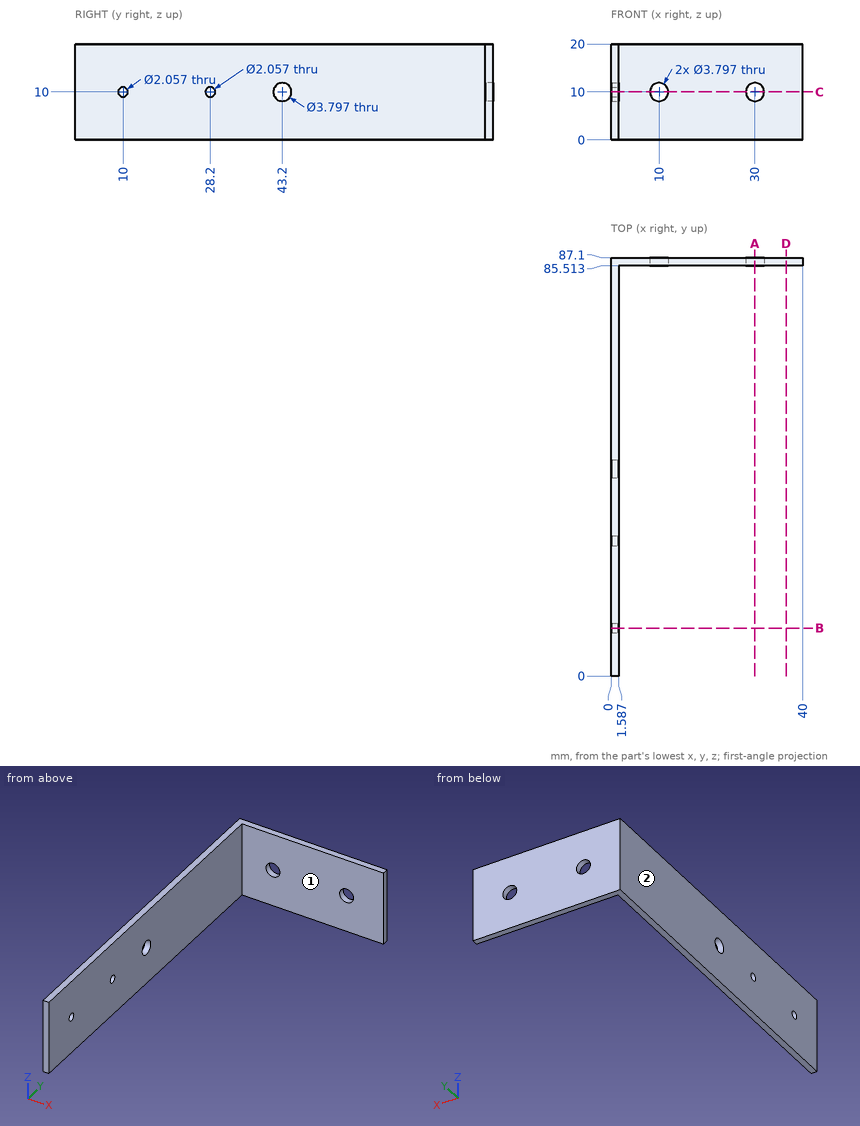
Check sheet for the drawn part. Datum: minimum x, y, z corner. Units: mm. A direction names the side the tool comes from. Coordinates: 2 decimals unless noted, no trailing zeros. Order: outer loops, then holes, each group sorted by start corner. A loop starts at its lowest first (then second) coordinate and runs counter-clockwise, first axis right, second up. Notation, with made-up numbers: M 69,-14 L 109,-14 A23 ccw 109,16 Z; hole C -26,15 d6. An arc over 180 degrees is marked long. One line per item, written item: value. Start each with the question number.
Item 1: Sectioned sample at B-B (y = 10). Enter the section's corners in (x, z).
Item 2: Access from +Z, -Z, +X, -X, +Y, -Y to the whole of each face (thin tool, end or side, straight path). Record for the marked faces 1 and 2.
Item 3: Sectioned sample at C-C (z = 10). Enter the section's corners in (x, y).
Item 4: Gauge pin test, flat ends, axial feed: pin 1 (5 mm diameter, centred on x = 27, z = 8, fed in from -Y); pin 2 (2.5 mm diameter, centred on y = 10, z = 10, fed in from +X). Record the tip position at first contact, or that the pin passes through.
Item 5: Sectioned sample at D-D (x = 36.5). Enter the section's corners in (y, z).
Item 6: Sectioned sample at A-A (x = 30). Enter the section's corners in (y, z).
Item 7: Scan lines: probe 1 along X at (y, z) = (86.45, 10); probe 2 along Y at (x, z) = (0.35, 10); probe 3 along Z at (x, y) = (10, 86). Record each from-to range of solid material in increasing order.
Conclusion:
1. outline: M 0,0 L 1.59,0 L 1.59,8.97 L 0,8.97 Z; M 0,11.03 L 1.59,11.03 L 1.59,20 L 0,20 Z
2. face 1: +Z, -Z, +X, -Y
2. face 2: +Z, -Z, -X, +Y, -Y
3. outline: M 0,0 L 1.59,0 L 1.59,8.97 L 0,8.97 Z; M 0,11.03 L 1.59,11.03 L 1.59,27.17 L 0,27.17 Z; M 0,29.23 L 1.59,29.23 L 1.59,41.3 L 0,41.3 Z; M 0,45.1 L 1.59,45.1 L 1.59,85.51 L 8.1,85.51 L 8.1,87.1 L 0,87.1 Z; M 11.9,85.51 L 28.1,85.51 L 28.1,87.1 L 11.9,87.1 Z; M 31.9,85.51 L 40,85.51 L 40,87.1 L 31.9,87.1 Z
4. pin 1: stops at y = 85.51
4. pin 2: stops at x = 1.59
5. outline: M 85.51,0 L 87.1,0 L 87.1,20 L 85.51,20 Z
6. outline: M 85.51,0 L 87.1,0 L 87.1,8.1 L 85.51,8.1 Z; M 85.51,11.9 L 87.1,11.9 L 87.1,20 L 85.51,20 Z
7. probe 1: x = 0 to 8.1, 11.9 to 28.1, 31.9 to 40
7. probe 2: y = 0 to 8.97, 11.03 to 27.17, 29.23 to 41.3, 45.1 to 87.1
7. probe 3: z = 0 to 8.1, 11.9 to 20
